from build123d import *

# Parameters (mm, degrees)
F1_DEPTH = 7
F3_DEPTH = 4


# Not quite as in the source:
# - a feature names something its author has since deleted; it is built from what else it names


with BuildPart() as f1:
    # F0 (on Top) → F1 (new body)
    with BuildSketch(Plane.XY):
        with BuildLine():
            Line((-19.6469386943, 23.4024446265), (-33.1021886284, 17.0788295944))
            Line((-33.1021886284, 17.0788295944), (-23.5166549683, -14.3096297979))
            ThreePointArc((-23.5166549683, -14.3096297979), (-19.5683456994, -21.0463448921), (-13.5673098266, -26.0423477739))
            Line((-13.5673098266, -26.0423477739), (2.2953252774, -35.1469367743))
            Line((2.2953252774, -35.1469367743), (3.609388601, -14.3096297979))
            ThreePointArc((3.609388601, -14.3096297979), (-2.48073947, -8.9765820448), (-5.2136145532, -1.3567098649))
            Line((-5.2136145532, -1.3567098649), (5.9560768355, 3.8057526561))
            Line((5.9560768355, 3.8057526561), (12.2448138941, 21.5456220774))
            Line((12.2448138941, 21.5456220774), (-8.0293232526, 12.2533091797))
            Line((-8.0293232526, 12.2533091797), (-6.2459499526, 15.5384703992))
            Line((-6.2459499526, 15.5384703992), (20.2230613727, 27.64663617))
            Line((20.2230613727, 27.64663617), (2.8586395134, 33.9794768895))
            Line((2.8586395134, 33.9794768895), (-10.5966104207, 27.6558618574))
            Line((-10.5966104207, 27.6558618574), (-15.1217745575, 25.529153242))
            Line((-15.1217745575, 25.529153242), (-19.6469386943, 23.4024446265))
        make_face()
        with BuildLine():
            Line((-21.966829896, -13.6883575469), (-31.0345193002, 16.6006959636))
            Line((-31.0345193002, 16.6006959636), (2.8586395134, 32.5295928335))
            Line((2.8586395134, 32.5295928335), (16.2475313521, 27.64663617))
            Line((16.2475313521, 27.64663617), (-13.5077397905, 14.0351812079))
            Line((-13.5077397905, 14.0351812079), (-19.4805990905, 19.85604316))
            Line((-19.4805990905, 19.85604316), (-18.8491754234, 11.0161071643))
            Line((-18.8491754234, 11.0161071643), (-27.2155441344, 7.2275632992))
            Line((-27.2155441344, 7.2275632992), (-18.0598944426, 5.6095388718))
            Line((-18.0598944426, 5.6095388718), (-17.3100791872, -3.1120055355))
            Line((-17.3100791872, -3.1120055355), (-12.5349350274, 4.6624024399))
            Line((-12.5349350274, 4.6624024399), (-3.5371426493, 3.3206269145))
            Line((-3.5371426493, 3.3206269145), (-9.4962064177, 9.7532588989))
            Line((-9.4962064177, 9.7532588989), (9.5593021267, 18.4870336848))
            Line((9.5593021267, 18.4870336848), (4.8924595123, 5.3223588356))
            Line((4.8924595123, 5.3223588356), (-7.6506364332, -0.4748705114))
            Line((-7.6506364332, -0.4748705114), (-5.8260546066, -7.0584053174))
            ThreePointArc((-5.8260546066, -7.0584053174), (-2.996906843, -12.2802585435), (1.8299611984, -15.7404858619))
            Line((1.8299611984, -15.7404858619), (0.7740783702, -32.4837844721))
            Line((0.7740783702, -32.4837844721), (-12.6359384992, -24.7869112046))
            ThreePointArc((-12.6359384992, -24.7869112046), (-18.2844119376, -20.0640956756), (-21.966829896, -13.6883575469))
        make_face(mode=Mode.SUBTRACT)
        with BuildLine():
            Line((-21.7736473098, 27.9276087633), (-19.6469386943, 23.4024446265))
            Line((-19.6469386943, 23.4024446265), (-15.1217745575, 25.529153242))
            Line((-15.1217745575, 25.529153242), (-10.5966104207, 27.6558618574))
            Line((-10.5966104207, 27.6558618574), (-12.7233190362, 32.1810259942))
            ThreePointArc((-12.7233190362, 32.1810259942), (-15.5525190095, 34.7579017095), (-19.3751917885, 34.5794815155))
            ThreePointArc((-19.3751917885, 34.5794815155), (-21.9520675037, 31.7502815423), (-21.7736473098, 27.9276087633))
        make_face()
        with BuildLine():
            ThreePointArc((-18.3118374807, 32.3168994471), (-14.9859011046, 31.1176716865), (-16.1851288653, 27.7917353104))
            ThreePointArc((-16.1851288653, 27.7917353104), (-19.5110652414, 28.990963071), (-18.3118374807, 32.3168994471))
        make_face(mode=Mode.SUBTRACT)
    extrude(amount=F1_DEPTH)

    # F2 (on face) → F3 (join)
    with BuildSketch(Plane(origin=(0, 0, 0), x_dir=(1, 0, 0), z_dir=(0, 0, -1))):
        with BuildLine():
            ThreePointArc((-12.6359384992, 24.7869112046), (-18.2844119376, 20.0640956756), (-21.966829896, 13.6883575469))
            Line((-21.966829896, 13.6883575469), (-31.0345193002, -16.6006959636))
            Line((-31.0345193002, -16.6006959636), (2.8586395134, -32.5295928335))
            Line((2.8586395134, -32.5295928335), (16.2475313521, -27.64663617))
            Line((16.2475313521, -27.64663617), (-13.5077397905, -14.0351812079))
            Line((-13.5077397905, -14.0351812079), (-19.4805990905, -19.85604316))
            Line((-19.4805990905, -19.85604316), (-18.8491754234, -11.0161071643))
            Line((-18.8491754234, -11.0161071643), (-27.2155441344, -7.2275632992))
            Line((-27.2155441344, -7.2275632992), (-18.0598944426, -5.6095388718))
            Line((-18.0598944426, -5.6095388718), (-17.3100791872, 3.1120055355))
            Line((-17.3100791872, 3.1120055355), (-12.5349350274, -4.6624024399))
            Line((-12.5349350274, -4.6624024399), (-3.5371426493, -3.3206269145))
            Line((-3.5371426493, -3.3206269145), (-9.4962064177, -9.7532588989))
            Line((-9.4962064177, -9.7532588989), (9.5593021267, -18.4870336848))
            Line((9.5593021267, -18.4870336848), (4.8924595123, -5.3223588356))
            Line((4.8924595123, -5.3223588356), (-7.6506364332, 0.4748705114))
            Line((-7.6506364332, 0.4748705114), (-5.8260546066, 7.0584053174))
            ThreePointArc((-5.8260546066, 7.0584053174), (-2.996906843, 12.2802585435), (1.8299611984, 15.7404858619))
            Line((1.8299611984, 15.7404858619), (0.7740783702, 32.4837844721))
            Line((0.7740783702, 32.4837844721), (-12.6359384992, 24.7869112046))
        make_face()
    extrude(amount=-F3_DEPTH)


solid = f1.part
Can you work these out from the model? Positions are in its coordinate system, mm. A direction names the side the tool comes from. Give positions to 0.01 mm unless a question says otherwise; leave off trailing zeros. Loops run counter-clockwise (first coordinate to the right, second up) from the corner with the lowest first, then second, coordinate; pieces in that order, holes last. Notation, with made-up numbers: (89.5, 47) -> (133.5, 47) arc R9 cw to (133.5, 63) -> close; hole circle Ø6 at (-15.75, -32.75). An arc over 180 degrees is marked (long way). Use one line per item in the form item = value.
1) I need wall thicknesses on line 1 along X through (y, z) = (8.5, 4.25); line 2 along Z through (x, y) = (5, 6); line 3 along Y through (x, z) = (14, 4.75). Which ranges of each line are inside material? Lowest first, please.
Answers:
line_1 = -30.48 to -28.61, -24.41 to -8.34, 6.02 to 7.62
line_2 = 0 to 4
line_3 = 24.8 to 26.62, 28.47 to 29.92
2) Will these pins go through, and if not, where does the flat tip stop? pin 1 (1 mm diameter, centred on x = -11, z = 5, fed in from +Y); pin 2 (3 mm diameter, centred on y = -17.5, z = 5, fed in from -X); pin 3 (5 mm diameter, centred on x = 2.5, y = 25.5, fed in from +Z).
Answers:
pin_1 = 29.58
pin_2 = -22.81
pin_3 = 4
3) If we section it at D-D (x = -2): Please give me the cut outline in (y, z).
Answers:
outline = (-32.68, 0) -> (-9.65, 0) -> (-9.65, 7) -> (-13.3, 7) -> (-13.3, 4) -> (-30.89, 4) -> (-30.89, 7) -> (-32.68, 7) -> close; (0.13, 0) -> (15.02, 0) -> (15.02, 7) -> (13.19, 7) -> (13.19, 4) -> (2.14, 4) -> (2.14, 7) -> (0.13, 7) -> close; (17.48, 0) -> (31.7, 0) -> (31.7, 7) -> (30.25, 7) -> (30.25, 4) -> (19.3, 4) -> (19.3, 7) -> (17.48, 7) -> close
4) If we section it at A-A (z = 1.5): Please give me the cut outline in (x, y), plus the area to 3 significant figures.
Answers:
outline = (-33.1, 17.08) -> (-23.52, -14.31) arc R22.65 ccw to (-13.57, -26.04) -> (2.3, -35.15) -> (3.61, -14.31) arc R16.13 cw to (-5.21, -1.36) -> (5.96, 3.81) -> (12.24, 21.55) -> (-8.03, 12.25) -> (-6.25, 15.54) -> (20.22, 27.65) -> (2.86, 33.98) -> (-10.6, 27.66) -> (-12.72, 32.18) arc R5 ccw to (-21.77, 27.93) -> (-19.65, 23.4) -> close; hole circle Ø5 at (-17.25, 30.05)
area = 1,800 mm²
5) We'd pull the mould along Y, two halves only. Please class faces 1 (the face through (11.66, 30.77, 3.45)), 2 (the face through (-28.377, 1.604, 3.451)), 3 (the face through (-20.725, 25.697, 3.451)): released by +Y, released by -Y, zero draft, split by the parting line, or undercut.
Answers:
face_1 = released by +Y
face_2 = released by -Y
face_3 = undercut
6) If we section it at C-C (y = 29.5): Please give me the cut outline in (x, z).
Answers:
outline = (-22.22, 0) -> (-19.69, 0) -> (-19.69, 7) -> (-22.22, 7) -> close; (-14.81, 0) -> (-11.46, 0) -> (-11.46, 7) -> (-14.81, 7) -> close; (-6.67, 0) -> (15.14, 0) -> (15.14, 7) -> (11.17, 7) -> (11.17, 4) -> (-3.59, 4) -> (-3.59, 7) -> (-6.67, 7) -> close
7) If we section it at B-B (y = 13): Please give me the cut outline in (x, z), plus the area to 3 significant figures.
Answers:
outline = (-31.86, 0) -> (-7.62, 0) -> (-7.62, 7) -> (-18.99, 7) -> (-18.99, 4) -> (-29.96, 4) -> (-29.96, 7) -> (-31.86, 7) -> close; (-6.4, 0) -> (9.22, 0) -> (9.22, 7) -> (7.61, 7) -> (7.61, 4) -> (-2.41, 4) -> (-2.41, 7) -> (-6.4, 7) -> close
area = 216 mm²
8) For faces 4 (the face through (6.803, 21.508, 3.451)), 5 (the face through (9.056, 12.552, 3.451)), 6 (the face through (-6.475, 6.492, 5.479)), which set-ups out of +Z, -Z, +X, -X, +Y, -Y let a thin tool reach every point of the face, with its end or its side?
Answers:
face_4 = +Z, -Z
face_5 = +Z, -Z, +X, -Y
face_6 = +Z
